Verification items for the finished model (mm, model axes). Face numbers are marked on the shaded views. A direction names the side the tool comes from. Give positions to 0.01 mm unless a question says otherwise; leave off trailing zeros. Order: outer loops, then holes, each group sorted by start corner. A loop starts at its lowest first (then second) coordinate and runs counter-clockwise, first axis right, second up.
from build123d import *

# Parameters (mm, degrees)
F0_W     = 165.1
F0_H     = 203.2
F1_DEPTH = 12.7
F3_D     = 14.2875
F3_DEPTH = 50.8
F3_TIP   = 4.2923980472
F4_W     = 330.2
F4_H     = 12.7
F5_DEPTH = 101.6
F6_SIZE  = 76.2
F7_SIZE  = 25.4


# Not quite as in the source:
# - a length typed as a fraction of an inch, garbled in the dataset ("3 / 203.2 mm" for 3/8 in), is restored


with BuildPart() as f1:
    # F0 (on Top) → F1 (new body)
    with BuildSketch(Plane.XY):
        Rectangle(F0_W, F0_H)
    extrude(amount=F1_DEPTH)

    # F3
    with Locations(Plane.XY.offset(12.7)):
        with Locations((-44.45, 76.2), (57.15, 76.2), (-44.45, -76.2), (57.15, -76.2)):
            Hole(F3_D / 2, depth=F3_DEPTH)
            with Locations((0, 0, -(F3_DEPTH + F3_TIP / 2))):  # 118° drill point
                Cone(0, F3_D / 2, F3_TIP, mode=Mode.SUBTRACT)

    # F4 (on face) → F5 (join)
    with BuildSketch(Plane(origin=(0, 0, 0), x_dir=(1, 0, 0), z_dir=(0, 0, -1))):
        with Locations((-82.55, 0)):
            Rectangle(F4_W, F4_H)
    extrude(amount=F5_DEPTH)

    # F6
    f6_edges = [f1.edges().sort_by_distance(p)[0] for p in [
        (82.55, 0, -101.6),
    ]]
    chamfer(f6_edges, length=F6_SIZE)

    # F7
    f7_edges = [f1.edges().sort_by_distance(p)[0] for p in [
        (-247.65, 0, 0),
    ]]
    chamfer(f7_edges, length=F7_SIZE)


solid = f1.part
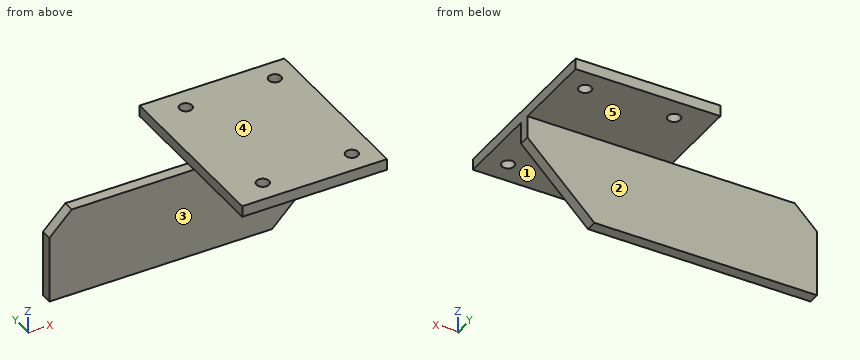
(1) Go/stop test with flat-tipped pins: pin 1 (2 mm diameter, centred on x = -204, z = -16.5, fed in from -Y); pin 2 (8 mm diameter, centred on x = -75.5, y = -64.5, fed in from -Z); pin 3 (12 mm diameter, centred on x = -166, z = -38, fed in from +Y). Record where each tip stops, or that it passes through.
Solved:
pin 1: stops at y = -6.35
pin 2: stops at z = 0
pin 3: stops at y = 6.35
(2) Section check B-B, the plane x = 57.15. Enter the section's corners in (y, z), then the cut area to 3 significant figures.
Solved:
outline: (-101.6, 0) - (-83.34, 0) - (-83.34, 12.7) - (-101.6, 12.7) - close; (-69.06, 0) - (-6.35, 0) - (-6.35, -50.8) - (6.35, -50.8) - (6.35, 0) - (69.06, 0) - (69.06, 12.7) - (-69.06, 12.7) - close; (83.34, 0) - (101.6, 0) - (101.6, 12.7) - (83.34, 12.7) - close
area: 2,860 mm2
(3) Section check C-C, the plane x = -44.45. Enter the section's corners in (y, z).
Solved:
outline: (-101.6, 0) - (-83.34, 0) - (-83.34, 12.7) - (-101.6, 12.7) - close; (-69.06, 0) - (-6.35, 0) - (-6.35, -101.6) - (6.35, -101.6) - (6.35, 0) - (69.06, 0) - (69.06, 12.7) - (-69.06, 12.7) - close; (83.34, 0) - (101.6, 0) - (101.6, 12.7) - (83.34, 12.7) - close
(4) Section check D-D, the plane z = -74. Enter the section's corners in (x, y).
Solved:
outline: (-247.65, -6.35) - (33.95, -6.35) - (33.95, 6.35) - (-247.65, 6.35) - close
(5) Scan lines: line 1 (Y direction, x = -44.45, z = 7.5); line 2 (X direction, y = 76, z = 3); line 3 (Z direction, x = 25, y = 31.5). Record each from-to range of solid material in increasing order.
Solved:
line 1: y = -101.6 to -83.34, -69.06 to 69.06, 83.34 to 101.6
line 2: x = -82.55 to -51.59, -37.31 to 50.01, 64.29 to 82.55
line 3: z = 0 to 12.7
(6) Release check for a two-part mould opening along Y. For the marked faces 1, 2 and 3 record: pulls with the +Y half, pulls with the -Y half, needs draft (parallel to the pull), parting line crosses it, or undercut.
Solved:
face 1: needs draft
face 2: pulls with the +Y half
face 3: pulls with the -Y half
(7) Section check A-A, the plane y = 76.2. Enter the section's corners in (x, z).
Solved:
outline: (-82.55, 0) - (-51.59, 0) - (-51.59, 12.7) - (-82.55, 12.7) - close; (-37.31, 0) - (50.01, 0) - (50.01, 12.7) - (-37.31, 12.7) - close; (64.29, 0) - (82.55, 0) - (82.55, 12.7) - (64.29, 12.7) - close
(8) Set-up check for the marked faces 4 and 5: record each of +Z, -Z, +X, -X, +Y, -Y from which the full face is reachable in a straight line by a thin tool's end or side.
Solved:
face 4: +Z, +X, -X, +Y, -Y
face 5: -Z, +X, -X, +Y
